from build123d import *

# Parameters (mm, degrees)
SKETCH1_W           = 100
SKETCH1_H           = 9
BOSS_EXTRUDE1_DEPTH = 5
CUT_EXTRUDE1_DEPTH  = 6
SKETCH3_W           = 20
SKETCH3_H           = 15
BOSS_EXTRUDE2_DEPTH = 9
SKETCH4_R           = 2.25
CUT_EXTRUDE2_DEPTH  = 10


with BuildPart() as part:
    # Sketch1 → Boss-Extrude1 (new body)
    with BuildSketch(Plane(origin=(0, 0, 0), x_dir=(1, 0, 0), z_dir=(0, 1, 0))):
        with Locations((50, 4.5)):
            Rectangle(SKETCH1_W, SKETCH1_H)
    extrude(amount=BOSS_EXTRUDE1_DEPTH)

    # Sketch2 → Cut-Extrude1 (cut, through all)
    with BuildSketch(Plane(origin=(0, 5, 0), x_dir=(1, 0, 0), z_dir=(0, 1, 0))):
        with BuildLine():
            Line((5, 6.25), (70, 6.25))
            ThreePointArc((70, 6.25), (71.75, 4.5), (70, 2.75))
            Line((70, 2.75), (5, 2.75))
            ThreePointArc((5, 2.75), (3.25, 4.5), (5, 6.25))
        make_face()
    extrude(amount=-CUT_EXTRUDE1_DEPTH, mode=Mode.SUBTRACT)

    # Sketch3 → Boss-Extrude2 (add)
    with BuildSketch(Plane(origin=(0, 0, -9), x_dir=(-1, 0, 0), z_dir=(0, 0, -1))):
        with Locations((-90, -2.5)):
            Rectangle(SKETCH3_W, SKETCH3_H)
    extrude(amount=-BOSS_EXTRUDE2_DEPTH)

    # Sketch4 → Cut-Extrude2 (cut)
    with BuildSketch(Plane(origin=(0, 0, -9), x_dir=(-1, 0, 0), z_dir=(0, 0, -1))):
        with BuildLine():
            Line((-100, 5), (-100, -2.5))
            ThreePointArc((-100, -2.5), (-97.803300859, 2.803300859), (-92.5, 5))
            Line((-92.5, 5), (-100, 5))
        make_face()
        with BuildLine():
            Line((-100, -10), (-92.5, -10))
            ThreePointArc((-92.5, -10), (-97.803300859, -7.803300859), (-100, -2.5))
            Line((-100, -2.5), (-100, -10))
        make_face()
        with Locations((-92.5, -2.5)):
            Circle(SKETCH4_R)
    extrude(amount=-CUT_EXTRUDE2_DEPTH, mode=Mode.SUBTRACT)


solid = part.part
Here's how the part is built. I have some questions about the finished solid (model axes, mm). A direction names the side the tool comes from. Coordinates: 2 decimals unless noted, no trailing zeros. Loops run counter-clockwise (first coordinate to the right, second up) from the corner with the lowest first, then second, coordinate; pieces in that order, holes last.
1. If we mould it in two halves opening along X, with no side actions, what happens to faces 1 (the flat face through (86, -10, -5)), 2 (the flat face through (37, 3, -6.25)), 3 (the flat face through (0, 2, -4))? For each: pulls with the +X half, pulls with the -X half, needs draft (parallel to the pull), parting line crosses it, or undercut.
2. I need wall thicknesses on L1, parallel to Z at x = 31, y = 2.5; L2, parallel to Y at x = 92.5, z = -1.75; L3, parallel to Y at x = 36, z = -6.5. Which ranges of each line are inside material? Lowest first, please.
3. For P1, Ø5, axis at x = 33, z = -5.5, coming from the -Y side; P2, Ø3.5, axis at x = 92.5, y = -2.5, coming from the -Z side; P3, Ø3, axis at y = -6, z = -8, coming from the +X side, each with a flat end and sliding along its axis, tell me the tip position at first contact or that it passes through.
4. Imagine slicing it at D-D, the plane x = 77. Please give me the cut outline in (y, z), and give its area (3 significant figures).
5. For faces 4 (the cylindrical face through (71.75, 2.54, -4.54)), 5 (the flat face through (80, -5, -5)), 6 (the flat face through (62, 1, 0)), which set-ups out of +Z, -Z, +X, -X, +Y, -Y let a thin tool reach every point of the face, with its end or its side?
6. Imagine slicing it at B-B, the plane x = 15.5. Please give me the cut outline in (y, z), and give its area (3 significant figures).
7. Imagine slicing it at C-C, the plane z = -1. Please give me the cut outline in (x, y), and give its area (3 significant figures).
8. Imagine slicing it at A-A, the plane z = -5. Please give me the cut outline in (x, y), and give its area (3 significant figures).
Taken from the geometry:
1. face 1: needs draft
1. face 2: undercut
1. face 3: pulls with the -X half
2. L1: z = -9 to -6.25, -2.75 to 0
2. L2: y = -10 to -4.75, -0.25 to 5
2. L3: y = 0 to 5
3. P1: stops at y = 0
3. P2: passes through
3. P3: stops at x = 99.73
4. outline: (0, -9) - (5, -9) - (5, 0) - (0, 0) - close
4. area: 45.0 mm2
5. face 4: +Y, -Y
5. face 5: +Z, -Z, -X, -Y
5. face 6: +Z, +X, -X, +Y, -Y
6. outline: (0, -9) - (5, -9) - (5, -6.25) - (0, -6.25) - close; (0, -2.75) - (5, -2.75) - (5, 0) - (0, 0) - close
6. area: 27.5 mm2
7. outline: (0, 0) - (80, 0) - (80, -10) - (92.5, -10) arc R7.5 ccw to (92.5, 5) - (0, 5) - close; hole circle Ø4.5 at (92.5, -2.5)
7. area: 660 mm2
8. outline: (0, 0) - (3.32, 0) - (3.32, 5) - (0, 5) - close; (71.68, 0) - (80, 0) - (80, -10) - (92.5, -10) arc R7.5 ccw to (92.5, 5) - (71.68, 5) - close; hole circle Ø4.5 at (92.5, -2.5)
8. area: 318 mm2
